from build123d import *

# Parameters (mm, degrees)
F1_DEPTH  = 203.2
F3_D      = 12.7
F8_DEPTH  = 381
F9_DEPTH  = 381
F10_DEPTH = 381
F11_DEPTH = 381


with BuildPart() as f1:
    # F0 (on Top) → F1 (new body)
    with BuildSketch(Plane.XY):
        with BuildLine():
            ThreePointArc((50.8, 44.45), (48.940128, 48.940128), (44.45, 50.8))
            Line((44.45, 50.8), (-44.45, 50.8))
            ThreePointArc((-44.45, 50.8), (-48.940128, 48.940128), (-50.8, 44.45))
            Line((-50.8, 44.45), (-50.8, -44.45))
            ThreePointArc((-50.8, -44.45), (-48.940128, -48.940128), (-44.45, -50.8))
            Line((-44.45, -50.8), (44.45, -50.8))
            ThreePointArc((44.45, -50.8), (48.940128, -48.940128), (50.8, -44.45))
            Line((50.8, -44.45), (50.8, 44.45))
        make_face()
        with BuildLine():
            ThreePointArc((44.45, 47.625), (46.695064, 46.695064), (47.625, 44.45))
            Line((47.625, 44.45), (47.625, -44.45))
            ThreePointArc((47.625, -44.45), (46.695064, -46.695064), (44.45, -47.625))
            Line((44.45, -47.625), (-44.45, -47.625))
            ThreePointArc((-44.45, -47.625), (-46.695064, -46.695064), (-47.625, -44.45))
            Line((-47.625, -44.45), (-47.625, 44.45))
            ThreePointArc((-47.625, 44.45), (-46.695064, 46.695064), (-44.45, 47.625))
            Line((-44.45, 47.625), (44.45, 47.625))
        make_face(mode=Mode.SUBTRACT)
    extrude(amount=F1_DEPTH)

    # F3 (through all)
    with Locations(Plane(origin=(-50.8, 0, 0), x_dir=(0, -1, 0), z_dir=(-1, 0, 0))):
        with Locations((0, 139.7)):
            Hole(F3_D / 2)

    # F7 (on face) → F8 (join)
    with BuildSketch(Plane.XZ.offset(50.8)):
        with BuildLine():
            Line((-31.430896, 0.929936), (-2.245064, 30.115768))
            ThreePointArc((-2.245064, 30.115768), (0, 31.045704), (2.245064, 30.115768))
            Line((2.245064, 30.115768), (31.430896, 0.929936))
            ThreePointArc((31.430896, 0.929936), (33.67596, 0), (35.921024, 0.929936))
            Line((35.921024, 0.929936), (0, 36.85096))
            Line((0, 36.85096), (-35.921024, 0.929936))
            ThreePointArc((-35.921024, 0.929936), (-33.67596, 0), (-31.430896, 0.929936))
        make_face()
    extrude(amount=F8_DEPTH)

    # F4 (on face) → F9 (join)
    with BuildSketch(Plane.YZ.offset(50.8)):
        with BuildLine():
            Line((35.921024, 0.929936), (0, 36.85096))
            Line((0, 36.85096), (-35.921024, 0.929936))
            ThreePointArc((-35.921024, 0.929936), (-34.89098, 0.241682), (-33.67596, 0))
            ThreePointArc((-33.67596, 0), (-32.460941, 0.241682), (-31.430896, 0.929936))
            Line((-31.430896, 0.929936), (-2.245064, 30.115768))
            ThreePointArc((-2.245064, 30.115768), (0, 31.045704), (2.245064, 30.115768))
            Line((2.245064, 30.115768), (31.430896, 0.929936))
            ThreePointArc((31.430896, 0.929936), (32.460941, 0.241682), (33.67596, 0))
            ThreePointArc((33.67596, 0), (34.89098, 0.241682), (35.921024, 0.929936))
        make_face()
    extrude(amount=F9_DEPTH)

    # F5 (on face) → F10 (join)
    with BuildSketch(Plane(origin=(0, 50.8, 0), x_dir=(-1, 0, 0), z_dir=(0, 1, 0))):
        with BuildLine():
            Line((35.921024, 0.929936), (0, 36.85096))
            Line((0, 36.85096), (-35.921024, 0.929936))
            ThreePointArc((-35.921024, 0.929936), (-34.89098, 0.241682), (-33.67596, 0))
            ThreePointArc((-33.67596, 0), (-32.460941, 0.241682), (-31.430896, 0.929936))
            Line((-31.430896, 0.929936), (-2.245064, 30.115768))
            ThreePointArc((-2.245064, 30.115768), (0, 31.045704), (2.245064, 30.115768))
            Line((2.245064, 30.115768), (31.430896, 0.929936))
            ThreePointArc((31.430896, 0.929936), (32.460941, 0.241682), (33.67596, 0))
            ThreePointArc((33.67596, 0), (34.89098, 0.241682), (35.921024, 0.929936))
        make_face()
    extrude(amount=F10_DEPTH)

    # F6 (on face) → F11 (join)
    with BuildSketch(Plane(origin=(-50.8, 0, 0), x_dir=(0, -1, 0), z_dir=(-1, 0, 0))):
        with BuildLine():
            Line((-31.430896, 0.929936), (-2.245064, 30.115768))
            ThreePointArc((-2.245064, 30.115768), (0, 31.045704), (2.245064, 30.115768))
            Line((2.245064, 30.115768), (31.430896, 0.929936))
            ThreePointArc((31.430896, 0.929936), (32.460941, 0.241682), (33.67596, 0))
            ThreePointArc((33.67596, 0), (34.89098, 0.241682), (35.921024, 0.929936))
            Line((35.921024, 0.929936), (0, 36.85096))
            Line((0, 36.85096), (-35.921024, 0.929936))
            ThreePointArc((-35.921024, 0.929936), (-34.89098, 0.241682), (-33.67596, 0))
            ThreePointArc((-33.67596, 0), (-32.460941, 0.241682), (-31.430896, 0.929936))
        make_face()
    extrude(amount=F11_DEPTH)


solid = f1.part
Can you work these out from the model? Positions are in its coordinate system, mm. A direction names the side the tool comes from. Coordinates: 2 decimals unless noted, no trailing zeros. Order: outer loops, then holes, each group sorted by start corner. A loop starts at its lowest first (then second) coordinate and runs counter-clockwise, first axis right, second up. Notation, with made-up numbers: M 7,-32.75 L 34,-32.75 A15 cw 34,-26.75 Z; hole C 17.25,39.5 d7. An arc over 180 degrees is marked long. Answer as CSV lines item,"result".
(1) Suppose I cut it at B-B on x = 96. Please give me the cut outline in (y, z) (3 decimals), plus the area to 3 significant figures.
Geometry check:
outline,"M -35.921,0.93 A3.175 ccw -33.676,0 A3.175 ccw -31.431,0.93 L -2.245,30.116 A3.175 cw 2.245,30.116 L 31.431,0.93 A3.175 ccw 33.676,0 A3.175 ccw 35.921,0.93 L 0,36.851 Z"
area,"310 mm^2"
(2) Suppose I cut it at A-A on z = 162. Please give me the cut outline in (x, y) (3 decimals), plus the area to 3 significant figures.
Geometry check:
outline,"M -50.8,-44.45 A6.35 ccw -44.45,-50.8 L 44.45,-50.8 A6.35 ccw 50.8,-44.45 L 50.8,44.45 A6.35 ccw 44.45,50.8 L -44.45,50.8 A6.35 ccw -50.8,44.45 Z; hole M -47.625,-44.45 A3.175 ccw -44.45,-47.625 L 44.45,-47.625 A3.175 ccw 47.625,-44.45 L 47.625,44.45 A3.175 ccw 44.45,47.625 L -44.45,47.625 A3.175 ccw -47.625,44.45 Z"
area,"1,220 mm^2"
(3) On a 3-axis mill with a long thin cutter (end or side, diameter ignored), from which of +Z, -Z, +X, -X, +Y, -Y can I reach the whole of each face in a straight line? I mean faces 1 (the flat face through (-18.21, 238.63, 18.64)), 2 (the flat face through (17.04, 238.63, 15.32)), 3 (the flat face through (-1, 47.625, 100)), 4 (the flat face through (238.63, -17.71, 19.14)). Say none if no direction works.
Geometry check:
face 1,"+Z, -X, +Y"
face 2,"-Z, +Y"
face 3,"+Z, -Z"
face 4,"+Z, +X, -Y"
(4) If we mould it in two halves opening along X, with no side actions, what happens to faces 5 (the flat face through (18.21, -238.63, 18.64)), 6 (the flat face through (47.625, 1, 100)), 7 (the flat face through (8, -431.8, 25))? For each: released by +X, released by -X, zero draft, split by the parting line, or undercut.
Geometry check:
face 5,"released by +X"
face 6,"undercut"
face 7,"zero draft"
(5) I'm going to push flat-ended pins straight in: pin 1 (3 mm diameter, centred on x = 184, z = 38, fed in from -Y); pin 2 (3 mm diameter, centred on y = -22, z = 149.5, fed in from -X); pin 3 (1 mm diameter, centred on x = -33.5, z = 47, fed in from -Y). Where does each tip first touch, or does it pass through?
Geometry check:
pin 1,"y = -0.35"
pin 2,"x = -50.8"
pin 3,"y = -50.8"
(6) Please list where these lines run through material, in increasing order: L1, parallel to Z at x = 49, y = 0; L2, parallel to X at y = 5, z = 51.5 (3 decimals); L3, parallel to Y at x = -223, z = 21.5.
Geometry check:
L1,"0 to 133.35, 146.05 to 203.2"
L2,"-50.8 to -47.625, 47.625 to 50.8"
L3,"-15.35 to -10.86, 10.86 to 15.35"
